Geometry check sheet. Reference: the model listing, model coordinates, mm. A direction names the side the tool comes from. Give positions to 0.01 mm unless a question says otherwise; leave off trailing zeros. Loops run counter-clockwise (first coordinate to the right, second up) from the corner with the lowest first, then second, coordinate; pieces in that order, holes last. Notation, with made-up numbers: (51.5, 16) -> (60.5, 16) arc R26 cw to (60.5, 47) -> close; hole circle Ø8 at (3, 53). An arc over 180 degrees is marked (long way). One line per item, written item: value. Start each with the question number.
(1) Gauge pin test, flat ends, axial feed: pin 1 Ø13.5 at (x, z) = (103.37, -43.82) entering from +Y; pin 2 Ø1.6 at (x, z) = (46.37, 61.18) entering from +Y; pin 3 Ø0.6 at (x, y) = (91.5, 1) entering from +Z; pin 4 Ø0.6 at (x, y) = (8.5, 1) entering from +Z. Record the tip position at first contact, or that the pin passes through.
(2) Draft check along X on faces 1 (the face through (63.31, 0.99, 12.42)), 2 (the face through (-103.76, 0.986, -39.675)), 3 (the face through (-62.9, 0.99, 11.33)), 4 (the face through (32.613, 0.986, -63.456)). Enter one of: pulls with the +X half, pulls with the -X half, needs draft (parallel to the pull), parting line crosses it, or undercut.
(3) Sectioned sample at C-C, the plane y = 1.55. State how many separate pieces and enclosed holes the cut face has, then the cut area to 3 significant figures.
(4) Tool access check on faces 5 (the face through (-1, 0, -44)), 6 (the face through (-54.895, 0.986, -5.755)). Record the directions out of +Z, -Z, +X, -X, +Y, -Y that give a thin tool (end or side, any length) a straight path to the whole face; none if there is none.
(5) Sectioned sample at A-A, the plane z = -1. Record the cut outline in (x, y).
(6) Sectioned sample at B-B, the plane x = 93.5. Record the cut outline in (y, z).
(7) Scan lines: line 1 along Z through (x, y) = (46, 0.1); line 2 along X through (y, z) = (1.6, 54); line 3 along Z through (x, y) = (-26, 0.85). Record each from-to range of solid material in increasing order. Write a range as from..to.
from build123d import *

# Parameters (mm, degrees)
SKETCH26_R          = 1
SKETCH26_R_2        = 2.15
SKETCH26_R_3        = 1.45
SKETCH26_R_4        = 4.25
SKETCH26_R_5        = 2.75
BOSS_EXTRUDE4_DEPTH = 2


with BuildPart() as part:
    # Sketch26 → Boss-Extrude4 (new body)
    with BuildSketch(Plane(origin=(0, 0, 0), x_dir=(1, 0, 0), z_dir=(0, 1, 0))):
        with BuildLine():
            Line((-20.823616498, -51.176455051), (21.352676296, -51.176455051))
            ThreePointArc((21.352676296, -51.176455051), (23.120443249, -51.908688098), (23.852676296, -53.676455051))
            Line((23.852676296, -53.676455051), (23.852676296, -73.676455051))
            ThreePointArc((23.852676296, -73.676455051), (24.584909343, -75.444222004), (26.352676296, -76.176455051))
            Line((26.352676296, -76.176455051), (48.872676296, -76.176455051))
            ThreePointArc((48.872676296, -76.176455051), (50.640443249, -75.444222004), (51.372676296, -73.676455051))
            Line((51.372676296, -73.676455051), (51.372676296, -51.552742091))
            ThreePointArc((51.372676296, -51.552742091), (51.400522432, -51.180646307), (51.483440514, -50.816839667))
            Line((51.483440514, -50.816839667), (75.469917209, 27.059447373))
            ThreePointArc((75.469917209, 27.059447373), (76.374187682, 28.334733163), (77.859152991, 28.823544949))
            Line((77.859152991, 28.823544949), (115.689249226, 28.823544949))
            ThreePointArc((115.689249226, 28.823544949), (117.457016179, 29.555777996), (118.189249226, 31.323544949))
            Line((118.189249226, 31.323544949), (118.189249226, 86.323544949))
            ThreePointArc((118.189249226, 86.323544949), (117.457016179, 88.091311902), (115.689249226, 88.823544949))
            Line((115.689249226, 88.823544949), (76.013272408, 88.823544949))
            Line((76.013272408, 88.823544949), (-75.48421261, 88.823544949))
            Line((-75.48421261, 88.823544949), (-76.032763958, 88.823544949))
            Line((-76.032763958, 88.823544949), (-115.160189428, 88.823544949))
            ThreePointArc((-115.160189428, 88.823544949), (-116.927956381, 88.091311902), (-117.660189428, 86.323544949))
            Line((-117.660189428, 86.323544949), (-117.660189428, 31.323544949))
            ThreePointArc((-117.660189428, 31.323544949), (-116.927956381, 29.555777996), (-115.160189428, 28.823544949))
            Line((-115.160189428, 28.823544949), (-77.320558078, 28.823544949))
            ThreePointArc((-77.320558078, 28.823544949), (-75.840570727, 28.338399148), (-74.934991096, 27.071254903))
            Line((-74.934991096, 27.071254903), (-50.523941264, -50.812146542))
            ThreePointArc((-50.523941264, -50.812146542), (-50.438282088, -51.18164852), (-50.409508246, -51.559856495))
            Line((-50.409508246, -51.559856495), (-50.409508246, -73.676455051))
            ThreePointArc((-50.409508246, -73.676455051), (-49.677275199, -75.444222004), (-47.909508246, -76.176455051))
            Line((-47.909508246, -76.176455051), (-25.823616498, -76.176455051))
            ThreePointArc((-25.823616498, -76.176455051), (-24.055849545, -75.444222004), (-23.323616498, -73.676455051))
            Line((-23.323616498, -73.676455051), (-23.323616498, -53.676455051))
            ThreePointArc((-23.323616498, -53.676455051), (-22.591383451, -51.908688098), (-20.823616498, -51.176455051))
        make_face()
        with Locations((-37.083616498, -71.176455051)):
            Circle(SKETCH26_R, mode=Mode.SUBTRACT)
        with Locations((-45.843616498, -61.176455051)):
            Circle(SKETCH26_R, mode=Mode.SUBTRACT)
        with Locations((-28.323616498, -61.176455051)):
            Circle(SKETCH26_R, mode=Mode.SUBTRACT)
        with BuildLine():
            Line((-43.378108588, -50.422722318), (-30.878108588, -50.422722318))
            ThreePointArc((-30.878108588, -50.422722318), (-30.128108588, -51.172722318), (-30.878108588, -51.922722318))
            Line((-30.878108588, -51.922722318), (-43.378108588, -51.922722318))
            ThreePointArc((-43.378108588, -51.922722318), (-44.128108588, -51.172722318), (-43.378108588, -50.422722318))
        make_face(mode=Mode.SUBTRACT)
        with Locations((-44.735470101, -37.176455051)):
            Circle(SKETCH26_R_2, mode=Mode.SUBTRACT)
        with Locations((-55.732763009, -11.697986619)):
            Circle(SKETCH26_R_3, mode=Mode.SUBTRACT)
        with Locations((-4.735470101, -6.176455051)):
            Circle(SKETCH26_R_2, mode=Mode.SUBTRACT)
        with Locations((28.852676296, -61.176455051)):
            Circle(SKETCH26_R, mode=Mode.SUBTRACT)
        with Locations((37.612676296, -71.176455051)):
            Circle(SKETCH26_R, mode=Mode.SUBTRACT)
        with Locations((46.372676296, -61.176455051)):
            Circle(SKETCH26_R, mode=Mode.SUBTRACT)
        with BuildLine():
            ThreePointArc((31.407168386, -51.922722318), (30.657168386, -51.172722318), (31.407168386, -50.422722318))
            Line((31.407168386, -50.422722318), (43.907168386, -50.422722318))
            ThreePointArc((43.907168386, -50.422722318), (44.657168386, -51.172722318), (43.907168386, -51.922722318))
            Line((43.907168386, -51.922722318), (31.407168386, -51.922722318))
        make_face(mode=Mode.SUBTRACT)
        with Locations((45.264529899, -37.176455051)):
            Circle(SKETCH26_R_2, mode=Mode.SUBTRACT)
        Polygon((35.712257561, -39.176455051), (-35.183197763, -39.176455051), (0.264529899, -20.951240159), align=None, mode=Mode.SUBTRACT)
        with Locations((5.264529899, -6.176455051)):
            Circle(SKETCH26_R_2, mode=Mode.SUBTRACT)
        with Locations((56.261822807, -11.697986619)):
            Circle(SKETCH26_R_3, mode=Mode.SUBTRACT)
        with Locations((-65.98606306, 21.76646972)):
            Circle(SKETCH26_R_3, mode=Mode.SUBTRACT)
        with Locations((-102.838209752, 43.823544949)):
            Circle(SKETCH26_R_4, mode=Mode.SUBTRACT)
        with BuildLine():
            ThreePointArc((-75.160005035, 39.191107079), (-75.910005035, 38.441107079), (-76.660005035, 39.191107079))
            Line((-76.660005035, 39.191107079), (-76.660005035, 51.691107079))
            ThreePointArc((-76.660005035, 51.691107079), (-75.910005035, 52.441107079), (-75.160005035, 51.691107079))
            Line((-75.160005035, 51.691107079), (-75.160005035, 39.191107079))
        make_face(mode=Mode.SUBTRACT)
        with Locations((-4.735470101, 42.323544949)):
            Circle(SKETCH26_R_2, mode=Mode.SUBTRACT)
        with Locations((-102.78421261, 63.123687889)):
            Circle(SKETCH26_R_3, mode=Mode.SUBTRACT)
        with Locations((-102.838212164, 73.323544949)):
            Circle(SKETCH26_R_5, mode=Mode.SUBTRACT)
        with Locations((-102.838214468, 83.523544949)):
            Circle(SKETCH26_R_3, mode=Mode.SUBTRACT)
        with Locations((-80.638212164, 73.323544949)):
            Circle(SKETCH26_R_3, mode=Mode.SUBTRACT)
        with BuildLine():
            ThreePointArc((-76.23421261, 81.095149015), (-75.48421261, 81.845149015), (-74.73421261, 81.095149015))
            Line((-74.73421261, 81.095149015), (-74.73421261, 68.595149015))
            ThreePointArc((-74.73421261, 68.595149015), (-75.48421261, 67.845149015), (-76.23421261, 68.595149015))
            Line((-76.23421261, 68.595149015), (-76.23421261, 81.095149015))
        make_face(mode=Mode.SUBTRACT)
        with Locations((-44.735470101, 52.823544949)):
            Circle(SKETCH26_R_2, mode=Mode.SUBTRACT)
        Polygon((-10.402901984, -2.176455051), (-46.543802783, -16.676455051), (-63.48421261, 28.823544949), (-63.48421261, 49.70968094), (-15.178445609, 38.323544949), (-0.735470101, 38.323544949), (-0.735470101, 42.323544949), (1.264529899, 42.323544949), (1.264529899, 38.323544949), (15.707505407, 38.323544949), (64.013272408, 49.70968094), (64.013272408, 28.823544949), (47.072862581, -16.676455051), (10.931961782, -2.176455051), (1.264529899, -2.176455051), (1.264529899, -6.176455051), (-0.735470101, -6.176455051), (-0.735470101, -2.176455051), align=None, mode=Mode.SUBTRACT)
        with Locations((5.264529899, 42.323544949)):
            Circle(SKETCH26_R_2, mode=Mode.SUBTRACT)
        with Locations((66.515122858, 21.76646972)):
            Circle(SKETCH26_R_3, mode=Mode.SUBTRACT)
        with BuildLine():
            Line((77.189064833, 51.691107079), (77.189064833, 39.191107079))
            ThreePointArc((77.189064833, 39.191107079), (76.439064833, 38.441107079), (75.689064833, 39.191107079))
            Line((75.689064833, 39.191107079), (75.689064833, 51.691107079))
            ThreePointArc((75.689064833, 51.691107079), (76.439064833, 52.441107079), (77.189064833, 51.691107079))
        make_face(mode=Mode.SUBTRACT)
        with Locations((103.367269549, 43.823544949)):
            Circle(SKETCH26_R_4, mode=Mode.SUBTRACT)
        Polygon((0.264529899, 49.70968094), (-63.538214468, 76.823544949), (64.067274266, 76.823544949), align=None, mode=Mode.SUBTRACT)
        with Locations((45.264529899, 52.823544949)):
            Circle(SKETCH26_R_2, mode=Mode.SUBTRACT)
        with Locations((103.313272408, 63.123687889)):
            Circle(SKETCH26_R_3, mode=Mode.SUBTRACT)
        with Locations((81.167271962, 73.323544949)):
            Circle(SKETCH26_R_3, mode=Mode.SUBTRACT)
        with BuildLine():
            Line((75.263272408, 68.595149015), (75.263272408, 81.095149015))
            ThreePointArc((75.263272408, 81.095149015), (76.013272408, 81.845149015), (76.763272408, 81.095149015))
            Line((76.763272408, 81.095149015), (76.763272408, 68.595149015))
            ThreePointArc((76.763272408, 68.595149015), (76.013272408, 67.845149015), (75.263272408, 68.595149015))
        make_face(mode=Mode.SUBTRACT)
        with Locations((103.367271962, 73.323544949)):
            Circle(SKETCH26_R_5, mode=Mode.SUBTRACT)
        with Locations((103.367274266, 83.523544949)):
            Circle(SKETCH26_R_3, mode=Mode.SUBTRACT)
    extrude(amount=BOSS_EXTRUDE4_DEPTH)


solid = part.part
Calculated:
1. pin 1: stops at y = 2
1. pin 2: passes through
1. pin 3: stops at z = -28.82
1. pin 4: stops at z = 51.18
2. face 1: pulls with the +X half
2. face 2: undercut
2. face 3: pulls with the -X half
2. face 4: undercut
3. separate pieces: 1
3. enclosed holes: 37
3. area: 16,800 mm2
4. face 5: +Z, -Z, +X, -X, -Y
4. face 6: +Y, -Y
5. outline: (-66.76, 0) -> (-53.13, 0) -> (-53.13, 2) -> (-66.76, 2) -> close; (53.65, 0) -> (67.44, 0) -> (67.44, 2) -> (53.65, 2) -> close
6. outline: (0, -88.82) -> (2, -88.82) -> (2, -28.82) -> (0, -28.82) -> close
7. line 1: z = -88.82..-76.82, -69.15..-54.84, -50.8..-45.46, 16.25..35.16, 39.2..60.25, 62.1..76.18
7. line 2: x = -50.41..-23.32, 23.85..51.37
7. line 3: z = -88.82..-76.82, -60.87..-40.87, 8.43..34.45, 39.18..76.18
